```python
from build123d import *

# Parameters (mm, degrees)
F1_DEPTH = 28
F2_R     = 1
F3_DEPTH = 25.5


with BuildPart() as f1:
    # F0 (on Front) → F1 (new body)
    with BuildSketch(Plane.XZ):
        with BuildLine():
            Line((8.25, 10.25), (-8.25, 10.25))
            ThreePointArc((-8.25, 10.25), (-9.6642135624, 9.6642135624), (-10.25, 8.25))
            Line((-10.25, 8.25), (-10.25, -8.25))
            ThreePointArc((-10.25, -8.25), (-9.6642135624, -9.6642135624), (-8.25, -10.25))
            Line((-8.25, -10.25), (8.25, -10.25))
            ThreePointArc((8.25, -10.25), (9.6642135624, -9.6642135624), (10.25, -8.25))
            Line((10.25, -8.25), (10.25, 8.25))
            ThreePointArc((10.25, 8.25), (9.6642135624, 9.6642135624), (8.25, 10.25))
        make_face()
        with BuildLine():
            ThreePointArc((-7.7, 6.7), (-8.4071067812, 8.4071067812), (-6.7, 7.7))
            Line((-6.7, 7.7), (6.7, 7.7))
            ThreePointArc((6.7, 7.7), (7.7, 8.7), (8.7, 7.7))
            ThreePointArc((8.7, 7.7), (8.4071067812, 6.9928932188), (7.7, 6.7))
            Line((7.7, 6.7), (7.7, -6.7))
            ThreePointArc((7.7, -6.7), (8.4071067812, -6.9928932188), (8.7, -7.7))
            ThreePointArc((8.7, -7.7), (7.7, -8.7), (6.7, -7.7))
            Line((6.7, -7.7), (-6.7, -7.7))
            ThreePointArc((-6.7, -7.7), (-8.4071067812, -8.4071067812), (-7.7, -6.7))
            Line((-7.7, -6.7), (-7.7, 6.7))
        make_face(mode=Mode.SUBTRACT)
        with BuildLine():
            Line((6.7, 7.7), (-6.7, 7.7))
            ThreePointArc((-6.7, 7.7), (-6.9928932188, 6.9928932188), (-7.7, 6.7))
            Line((-7.7, 6.7), (-7.7, -6.7))
            ThreePointArc((-7.7, -6.7), (-6.9928932188, -6.9928932188), (-6.7, -7.7))
            Line((-6.7, -7.7), (6.7, -7.7))
            ThreePointArc((6.7, -7.7), (6.9928932188, -6.9928932188), (7.7, -6.7))
            Line((7.7, -6.7), (7.7, 6.7))
            ThreePointArc((7.7, 6.7), (6.9928932188, 6.9928932188), (6.7, 7.7))
        make_face()
    extrude(amount=F1_DEPTH)

    # F2 (on face) → F3 (join)
    with BuildSketch(Plane.XZ.offset(28)):
        with Locations((-7.7, 7.7)):
            Circle(F2_R)
        with Locations((7.7, 7.7)):
            Circle(F2_R)
        with Locations((7.7, -7.7)):
            Circle(F2_R)
        with Locations((-7.7, -7.7)):
            Circle(F2_R)
    extrude(amount=-F3_DEPTH)

    # F5 (on offset) → F6 (revolve)
    with BuildSketch(Plane(origin=(0, 0, 0), x_dir=(0, -1, 0), z_dir=(-1, 0, 0))):
        Polygon((-10, 0), (0, 0), (0, 8), (-1.5, 8), (-1.5, 2), (-10, 2), align=None)
    revolve(axis=Axis((0, 5, 0), (0, 1, 0)))


solid = f1.part
```
Input: part model. Units: mm. Frame: model coordinates. A direction names the side the tool comes from. Give positions to 0.01 mm unless a question says otherwise; leave off trailing zeros. Order: outer loops, then holes, each group sorted by start corner. A loop starts at its lowest first (then second) coordinate and runs counter-clockwise, first axis right, second up. Notation, with made-up numbers: M 1.25,37 L 41.25,37 A13 ccw 41.25,61 Z; hole C -35.5,50 d9. An arc over 180 degrees is marked long. One line per question, with ' | ' between items. Start each with the question number.
1. Pull-direction query (Z, two-part tool) for faces 1 (the face through (-2, 1.5, 2)), 2 (the face through (0, -14, -10.25)), 3 (the face through (-8, -2.5, -8)), 4 (the face through (-9.65, -13.8, 9.68)); classes: released by +Z, released by -Z, zero draft, split by the parting line, or undercut.
2. First-contact query: pin 1 Ø1.5 at (y, z) = (5.5, -1) entering from -X; pin 2 Ø1.6 at (x, z) = (8, -7.5) entering from +Y; pin 3 Ø12 at (x, z) = (6.5, -5) entering from +Y. Flat tips, straight axial feed; report the tip coordinate or a pass-through.
3. Section query A-A (z = 0). Return the cut outline in (x, y).
4. Section query C-C (y = 5.5). Return the cut outline in (x, z), and give its area (3 significant figures).
5. Material intervals for probe 1 along X at (y, z) = (-0.6, -7.7); probe 2 along Y at (x, z) = (8.5, 3.25); probe 3 along Y at (x, z) = (-5.5, -0.5), sorted ascending. Write a range as [from, to].
6. Section query D-D (x = 5). Return the cut outline in (y, z) (3 decimals).
7. Access query for faces 5 (the face through (4.4, 0, 7)), 6 (the face through (10.25, -14, 0)). Directions: +Z, -Z, +X, -X, +Y, -Y. A direction counts if a zero-diameter tool reaches every point of the face in a straight line with its end or side. Return the directions, or none.
8. Section query B-B (x = 0). Return the cut outline in (y, z).
Here are the results:
1) face 1: zero draft | face 2: released by -Z | face 3: undercut | face 4: released by +Z
2) pin 1: x = -1.98 | pin 2: y = 0 | pin 3: y = 1.5
3) outline: M -10.25,-28 L 10.25,-28 L 10.25,0 L 8,0 L 8,1.5 L 2,1.5 L 2,10 L -2,10 L -2,1.5 L -8,1.5 L -8,0 L -10.25,0 Z
4) outline: C 0,0 d4 | area: 12.6 mm²
5) probe 1: [-10.25, -8.7], [-6.7, 6.7], [8.7, 10.25] | probe 2: [-28, 0] | probe 3: [-28, 1.5]
6) outline: M -28,-10.25 L 0,-10.25 L 0,-6.245 L 1.5,-6.245 L 1.5,6.245 L 0,6.245 L 0,10.25 L -28,10.25 Z
7) face 5: +Y | face 6: +Z, -Z, +X, +Y, -Y
8) outline: M -28,-10.25 L 0,-10.25 L 0,-8 L 1.5,-8 L 1.5,-2 L 10,-2 L 10,2 L 1.5,2 L 1.5,8 L 0,8 L 0,10.25 L -28,10.25 Z
